Autodesk Inventor part; units mm, degrees
ref_plane "YZ Plane" through (0, 0, 0) normal (1, 0, 0) x (0, 1, 0)
ref_plane "XZ Plane" through (0, 0, 0) normal (0, 1, 0) x (-1, 0, 0)
ref_plane "XY Plane" through (0, 0, 0) normal (0, 0, 1) x (1, 0, 0)
sketch "Esquisse2" plane through (0, 0, 0) normal (0, 0, 1) x (1, 0, 0)
  line L0 (-78.4497, 0) -> (78.4497, 0) construction
  line L1 (0, -64.4497) -> (0, 64.4497) construction
  line L2 (-50, -45) -> (50, -45)
  line L3 (55, -40) -> (55, 40)
  line L4 (50, 45) -> (-50, 45)
  line L5 (-55, 40) -> (-55, -40)
  line L6 (-55, -45) -> (55, 45) construction
  line L7 (55, -45) -> (-55, 45) construction
  arc A0 (-50, 45) -> (-55, 40) centre (-50, 40) ccw
  arc A1 (-55, -40) -> (-50, -45) centre (-50, -40) ccw
  arc A2 (50, -45) -> (55, -40) centre (50, -40) ccw
  arc A3 (55, 40) -> (50, 45) centre (50, 40) ccw
  point P0 (0, 0)
  dimension "d0" = 110
  dimension "d1" = 90
  dimension "d2" = 5
extrude "Extrusion1" add sketch "Esquisse2" along normal blind 8
fillet "Congé1" radius 4 8 edges at (53.5355, -43.5355, 8) (55, 0, 8) (53.5355, 43.5355, 8) (0, 45, 8) (-53.5355, 43.5355, 8) (-55, 0, 8) (-53.5355, -43.5355, 8) (0, -45, 8)
sketch "Esquisse3" plane through (0, 0, 8) normal (0, 0, 1) x (1, 0, 0)
  line L0 (-83, 0) -> (78, 0) construction
  line L1 (0, -64) -> (0, 69) construction
  line L2 (50, 45) -> (-50, 45) construction
  line L3 (-55, 40) -> (-55, -40) construction
  line L4 (-55, 45) -> (-26, 45) construction
  line L5 (-26, 45) -> (-26, 30) construction
  line L6 (-26, 30) -> (-55, 30) construction
  line L7 (-55, 30) -> (-55, 45) construction
  line L8 (-26, 30) -> (26.5, 30)
  line L9 (26.5, 30) -> (26.5, -10)
  line L10 (26.5, -10) -> (-26, -10)
  line L11 (-26, -10) -> (-26, 30)
  point P0 (0, 0)
  dimension "d6" = 29
  dimension "d7" = 15
  dimension "d8" = 52.5
  dimension "d9" = 40
extrude "Extrusion2" cut sketch "Esquisse3" against normal through all
sketch "Esquisse4" plane through (0, 0, 0) normal (0, 0, -1) x (-1, 0, 0)
  line L0 (0, -71.6569) -> (0, 72.6924) construction
  line L1 (86.6924, 0) -> (-85.6569, 0) construction
  line L2 (-50.5, -42.5) -> (50.5, -42.5)
  line L3 (52.5, -40.5) -> (52.5, 40.5)
  line L4 (50.5, 42.5) -> (-50.5, 42.5)
  line L5 (-52.5, 40.5) -> (-52.5, -40.5)
  line L6 (-52.5, -42.5) -> (52.5, 42.5) construction
  line L7 (52.5, -42.5) -> (-52.5, 42.5) construction
  arc A0 (-50.5, 42.5) -> (-52.5, 40.5) centre (-50.5, 40.5) ccw
  arc A1 (-52.5, -40.5) -> (-50.5, -42.5) centre (-50.5, -40.5) ccw
  arc A2 (50.5, -42.5) -> (52.5, -40.5) centre (50.5, -40.5) ccw
  arc A3 (52.5, 40.5) -> (50.5, 42.5) centre (50.5, 40.5) ccw
  line L8 (-26.5, -10) -> (-26.5, 30) construction
  line L9 (-26.5, 30) -> (26, 30) construction
  line L10 (26, 30) -> (26, -10) construction
  line L11 (26, -10) -> (-26.5, -10) construction
  arc A4 (50, -45) -> (55, -40) centre (50, -40) ccw construction
  line L12 (55, 40) -> (55, -40) construction
  arc A5 (55, 40) -> (50, 45) centre (50, 40) ccw construction
  line L13 (-50, 45) -> (50, 45) construction
  arc A6 (-50, 45) -> (-55, 40) centre (-50, 40) ccw construction
  line L14 (-55, -40) -> (-55, 40) construction
  arc A7 (-55, -40) -> (-50, -45) centre (-50, -40) ccw construction
  line L15 (50, -45) -> (-50, -45) construction
  line L16 (55, 40) -> (55, -40) construction
  line L17 (-50, 45) -> (50, 45) construction
  point P0 (0, 0)
  dimension "d12" = 105
  dimension "d13" = 85
  dimension "d14" = 2
extrude "Extrusion3" cut sketch "Esquisse4" against normal blind 6
sketch "Esquisse5" plane through (0, 0, 0) normal (0, 0, -1) x (-1, 0, 0)
  line L0 (0, -71.6569) -> (0, 72.6924) construction
  line L1 (85.6569, 0) -> (-86.6924, 0) construction
  line L2 (-52.5, -40.5) -> (-52.5, 40.5) construction
  arc A0 (-50.5, 42.5) -> (-52.5, 40.5) centre (-50.5, 40.5) ccw construction
  line L3 (-50.5, 42.5) -> (50.5, 42.5) construction
  arc A1 (52.5, 40.5) -> (50.5, 42.5) centre (50.5, 40.5) ccw construction
  line L4 (52.5, 40.5) -> (52.5, -40.5) construction
  arc A2 (50.5, -42.5) -> (52.5, -40.5) centre (50.5, -40.5) ccw construction
  line L5 (50.5, -42.5) -> (-50.5, -42.5) construction
  arc A3 (-52.5, -40.5) -> (-50.5, -42.5) centre (-50.5, -40.5) ccw construction
  arc A4 (50, -45) -> (55, -40) centre (50, -40) ccw construction
  line L6 (55, 40) -> (55, -40) construction
  arc A5 (55, 40) -> (50, 45) centre (50, 40) ccw construction
  line L7 (-50, 45) -> (50, 45) construction
  arc A6 (-50, 45) -> (-55, 40) centre (-50, 40) ccw construction
  line L8 (-55, -40) -> (-55, 40) construction
  arc A7 (-55, -40) -> (-50, -45) centre (-50, -40) ccw construction
  line L9 (50, -45) -> (-50, -45) construction
  line L10 (-55, 45) -> (-35, 45) construction
  line L11 (-35, 45) -> (-35, 42.5) construction
  line L12 (-35, 42.5) -> (-55, 42.5) construction
  line L13 (-55, 42.5) -> (-55, 45) construction
  line L14 (-55, -40) -> (-55, 40) construction
  line L15 (-50, 45) -> (50, 45) construction
  line L16 (-35, 42.5) -> (-25, 42.5)
  line L17 (-25, 42.5) -> (-25, 43.5)
  line L18 (-25, 43.5) -> (-35, 43.5)
  line L19 (-35, 43.5) -> (-35, 42.5)
  point P0 (0, 0)
  dimension "d17" = 20
  dimension "d18" = 2.5
  dimension "d19" = 10
  dimension "d20" = 1
extrude "Extrusion4" add sketch "Esquisse5" along normal blind 6
sketch "Esquisse6" plane through (25, 43.5, 0) normal (0, 1, 0) x (1, 0, 0)
  line L0 (10, 0) -> (0, 0) construction
  line L1 (10, 0) -> (10, 6) construction
  line L2 (0, 6) -> (10, 6) construction
  line L3 (0, 0) -> (0, 6) construction
  line L4 (0, 6) -> (10, 6)
  line L5 (10, 6) -> (10, 3)
  line L6 (10, 3) -> (0, 3)
  line L7 (0, 3) -> (0, 6)
  point P0 (-25, 0)
  dimension "d23" = 3
extrude "Extrusion5" add sketch "Esquisse6" along normal blind 0.5
mirror "Symétrie1" about plane through (0, 0, 0) normal (1, 0, 0) of "Extrusion4", "Extrusion5"
mirror "Symétrie2" about plane through (0, 0, 0) normal (0, 1, 0) of "Extrusion4", "Extrusion5", "Symétrie1"
chamfer "Chanfrein1" distance 2.5 angle 25 1 edges at (30, 44, -6) measured on face at (28.3333, 44, -5)
sketch "Esquisse9" plane through (0, 0, 6) normal (0, 0, -1) x (-1, 0, 0)
  line L0 (35, -42.5) -> (35, -43.5) construction
  line L1 (25, -43.5) -> (25, -42.5) construction
  line L2 (-25, -42.5) -> (-25, -43.5) construction
  line L3 (-35, -43.5) -> (-35, -42.5) construction
  line L4 (25, 42.5) -> (25, 43.5) construction
  line L5 (35, 43.5) -> (35, 42.5) construction
  line L6 (-35, 42.5) -> (-35, 43.5) construction
  line L7 (-25, 43.5) -> (-25, 42.5) construction
  arc A0 (52.5, 40.5) -> (50.5, 42.5) centre (50.5, 40.5) ccw construction
  line L8 (52.5, 40.5) -> (52.5, -40.5) construction
  arc A1 (50.5, -42.5) -> (52.5, -40.5) centre (50.5, -40.5) ccw construction
  line L9 (50.5, -42.5) -> (35, -42.5) construction
  arc A2 (-52.5, -40.5) -> (-50.5, -42.5) centre (-50.5, -40.5) ccw construction
  line L10 (-52.5, -40.5) -> (-52.5, 40.5) construction
  arc A3 (-50.5, 42.5) -> (-52.5, 40.5) centre (-50.5, 40.5) ccw construction
  line L11 (-50.5, 42.5) -> (-35, 42.5) construction
  arc A4 (50, -45) -> (55, -40) centre (50, -40) ccw construction
  line L12 (55, 40) -> (55, -40) construction
  arc A5 (55, 40) -> (50, 45) centre (50, 40) ccw construction
  line L13 (-50, 45) -> (50, 45) construction
  arc A6 (-50, 45) -> (-55, 40) centre (-50, 40) ccw construction
  line L14 (-55, -40) -> (-55, 40) construction
  arc A7 (-55, -40) -> (-50, -45) centre (-50, -40) ccw construction
  line L15 (50, -45) -> (-50, -45) construction
  line L16 (55, 40) -> (55, -40) construction
  line L17 (-50, 45) -> (50, 45) construction
  circle A8 centre (35, 35) radius 4
  line L18 (78.4497, 0) -> (-78.4497, 0) construction
  line L19 (0, -64.4497) -> (0, 64.4497) construction
  line L20 (0, 0) -> (35, 0) construction
  line L21 (35, 0) -> (35, 35) construction
  line L22 (35, 35) -> (0, 35) construction
  line L23 (0, 35) -> (0, 0) construction
  line L24 (35, -43.5) -> (25, -43.5)
  line L25 (-25, -43.5) -> (-35, -43.5)
  line L26 (25, 43.5) -> (35, 43.5)
  line L27 (-35, 43.5) -> (-25, 43.5)
  line L28 (25, -42.5) -> (-25, -42.5)
  line L29 (-35, -42.5) -> (-50.5, -42.5)
  line L30 (-25, 42.5) -> (25, 42.5)
  line L31 (35, 42.5) -> (50.5, 42.5)
  dimension "d49" = 8
  dimension "d52" = 35
  dimension "d53" = 35
extrude "Extrusion7" add sketch "Esquisse9" along normal blind 4
sketch "Esquisse7" plane through (0, 0, 8) normal (0, 0, 1) x (1, 0, 0)
  circle A0 centre (-44, 19.5) radius 5
  circle A1 centre (-35, 35) radius 2.7
  line L0 (0, 0) -> (-35, 0) construction
  line L1 (-35, 0) -> (-35, 35) construction
  line L2 (-35, 35) -> (0, 35) construction
  line L3 (0, 35) -> (0, 0) construction
  line L4 (-35, 35) -> (-37.15, 35) construction
  line L5 (-37.15, 33.3668) -> (-37.15, 36.6332)
  line L6 (-32.85, 33.3668) -> (-32.85, 36.6332)
  line L7 (0, 0) -> (-44, 0) construction
  line L8 (-44, 0) -> (-44, 19.5) construction
  line L9 (-44, 19.5) -> (0, 19.5) construction
  line L10 (0, 19.5) -> (0, 0) construction
  dimension "d34" = 10
  dimension "d39" = 5.4
  dimension "d54" = 35
  dimension "d55" = 35
  dimension "d56" = 2.15
  dimension "d57" = 44
  dimension "d58" = 19.5
extrude "Extrusion6" cut sketch "Esquisse7" against normal through all contours A0 | L6 A1 L5
sketch "Esquisse11" plane through (0, 0, 8) normal (0, 0, 1) x (1, 0, 0)
  point P0 (0, 0)
chamfer "Chanfrein3" distance 2.5 angle 25 1 edges at (-30, 44, -6) measured on face at (-28.3333, 44, -5)
chamfer "Chanfrein4" distance 2.5 angle 25 1 edges at (-30, -44, -6) measured on face at (-28.3333, -44, -5)
chamfer "Chanfrein5" distance 2.5 angle 25 1 edges at (30, -44, -6) measured on face at (28.3333, -44, -5)
properties part number "_Impression 3D"
Here's how the part is built. I have some questions about the finished solid (model axes, mm). A direction names the side the tool comes from. Give positions to 0.01 mm unless a question says otherwise; leave off trailing zeros. Order: outer loops, then holes, each group sorted by start corner. A loop starts at its lowest first (then second) coordinate and runs counter-clockwise, first axis right, second up. Notation, with made-up numbers: (33, 8) - (76, 8) arc R16 cw to (76, 20) - close; hole circle Ø10 at (15, 47). An arc over 180 degrees is marked (long way). Answer as a JSON object with one key per item and string values. Group by question number.
Item 1: For P1, Ø1.5, axis at x = -29, z = -1.5, coming from the -Y side; P2, Ø0.6, axis at x = -30.5, y = 43.5, coming from the +Z side; P3, Ø1.6, axis at y = 3, z = 6.5, coming from the -X side; P4, Ø8, axis at x = -16, y = -3.5, coming from the +Z side, each with a flat end and sliding along its axis, tell me the tip position at first contact or that it passes through.
Item 2: If we section it at D-D on x = 33.5: Please give me the cut outline in (y, z), and give its area (3 significant figures).
Item 3: If we section it at A-A on x = -44: Please give me the cut outline in (y, z).
Item 4: If we mould it in two halves opening along X, with no side actions, what happens to faces 6 (the flat face through (-38, 35, 2)), 7 (the flat face through (-30, 43.5, -1)), 8 (the cylindrical face through (-53, -44, 2))? For each: pulls with the +X half, pulls with the -X half, needs draft (parallel to the pull), parting line crosses it, or undercut.
Item 5: If we section it at C-C on y = 35: Please give me the cut outline in (x, z).
Item 6: Which directions (+Z, -Z, +X, -X, +Y, -Y) give clear straight access to the entire face, cutting with the end or side of a thin tool? Please do faces 1 (the flat face through (30, -43.5, -1)), 2 (the flat face through (55, -1, 2)), 3 (the cylindrical face through (53, 44, 2)), 4 (the flat face through (30, 43.5, -1)), 5 (the flat face through (-1, 42.5, 3)).
Item 7: Please list where these lines run through material, in increasing order: probe 1 along Y at (x, z) = (-44, 7.1); probe 2 along Y at (x, z) = (-42, 1); probe 3 along Z at (x, y) = (-34.5, 15).
Item 8: If we section it at B-B on y = 19.5: Please give me the cut outline in (x, z), and give its area (3 significant figures).
Result set:
{
 "1": {"P1": "y = -43.5", "P2": "z = 7.34", "P3": "x = -54.62", "P4": "through"},
 "2": {"outline": "(-45, 0) - (-43.5, 0) - (-43.5, -3) - (-44, -3) - (-44, -3.5) - (-42.83, -6) - (-42.5, -6) - (-42.5, 6) - (42.5, 6) - (42.5, -6) - (42.83, -6) - (44, -3.5) - (44, -3) - (43.5, -3) - (43.5, 0) - (45, 0) - (45, 4) arc R4 ccw to (41, 8) - (-41, 8) arc R4 ccw to (-45, 4) - close", "area": "215 mm²"},
 "3": {"outline": "(-45, 0) - (-42.5, 0) - (-42.5, 6) - (14.5, 6) - (14.5, 8) - (-41, 8) arc R4 ccw to (-45, 4) - close; (24.5, 6) - (42.5, 6) - (42.5, 0) - (45, 0) - (45, 4) arc R4 ccw to (41, 8) - (24.5, 8) - close"},
 "4": {"face 6": "undercut", "face 7": "needs draft", "face 8": "pulls with the -X half"},
 "5": {"outline": "(-55, 0) - (-52.5, 0) - (-52.5, 6) - (-39, 6) - (-39, 2) - (-37.15, 2) - (-37.15, 8) - (-51, 8) arc R4 ccw to (-55, 4) - close; (-32.85, 2) - (-31, 2) - (-31, 6) - (52.5, 6) - (52.5, 0) - (55, 0) - (55, 4) arc R4 ccw to (51, 8) - (-32.85, 8) - close"},
 "6": {"face 1": "+X, -X, -Y", "face 2": "+Z, -Z, +X, +Y, -Y", "face 3": "+Z, -Z, +X, +Y", "face 4": "+X, -X, +Y", "face 5": "-Z"},
 "7": {"probe 1": "-43.53 to 14.5, 24.5 to 43.53", "probe 2": "-45 to -42.5, 42.5 to 45", "probe 3": "6 to 8"},
 "8": {"outline": "(-55, 0) - (-52.5, 0) - (-52.5, 6) - (-49, 6) - (-49, 8) - (-51, 8) arc R4 ccw to (-55, 4) - close; (-39, 6) - (-26, 6) - (-26, 8) - (-39, 8) - close; (26.5, 6) - (52.5, 6) - (52.5, 0) - (55, 0) - (55, 4) arc R4 ccw to (51, 8) - (26.5, 8) - close", "area": "118 mm²"}
}
